from build123d import *

# Parameters (mm, degrees)
PAD001_DEPTH    = 30
POCKET002_DEPTH = 15
SKETCH010_R     = 2.951076
SKETCH010_W     = 16.720002
SKETCH010_H     = 13.459998
POCKET003_DEPTH = 5
SKETCH011_R     = 3.068583
SKETCH011_W     = 16.509998
SKETCH011_H     = 13.460002
POCKET004_DEPTH = 5


with BuildPart() as part:
    # Sketch008 → Pad001 (new body, symmetric)
    with BuildSketch(Plane.YZ):
        Polygon((-37.5, 10), (37.5, 10), (37.5, 30.376934), (-10.046035, 30.376934), align=None)
    extrude(amount=PAD001_DEPTH, both=True)

    # Sketch009 (on Face1 of Pad001) → Pocket002 (cut)
    with BuildSketch(Plane.YX.offset(-10)):
        with BuildLine():
            Line((-16.668194, 25.274987), (-16.668194, -26.160018))
            ThreePointArc((-16.668194, -26.160018), (-15.924248, -27.956072), (-14.128194, -28.700018))
            Line((-14.128194, -28.700018), (31.591806, -28.700018))
            ThreePointArc((31.591806, -28.700018), (33.387861, -27.956083), (34.131806, -26.160032))
            Line((34.131806, -26.160032), (34.131806, 25.909982))
            ThreePointArc((34.131806, 25.909982), (33.38786, 27.706037), (31.591806, 28.449982))
            Line((-13.493194, 28.449982), (31.591806, 28.449982))
            ThreePointArc((-13.493194, 28.449982), (-15.738253, 27.520045), (-16.668194, 25.274987))
        make_face()
    extrude(amount=-POCKET002_DEPTH, mode=Mode.SUBTRACT)

    # Sketch010 (on Face3 of Pocket002) → Pocket003 (cut)
    with BuildSketch(Plane(origin=(-30, 0, 0), x_dir=(0, 1, 0), z_dir=(-1, 0, 0))):
        with Locations((-9.634073, -10.729566)):
            Circle(SKETCH010_R)
        with Locations((19.018807, -14.92554)):
            Rectangle(SKETCH010_W, SKETCH010_H)
    extrude(amount=-POCKET003_DEPTH, mode=Mode.SUBTRACT)

    # Sketch011 (on Face14 of Pocket003) → Pocket004 (cut)
    with BuildSketch(Plane.YZ.offset(30)):
        with Locations((3.356387, 11.259916)):
            Circle(SKETCH011_R)
        with Locations((-9.699885, 11.221059)):
            Circle(SKETCH011_R)
        with Locations((18.913807, 14.92554)):
            Rectangle(SKETCH011_W, SKETCH011_H)
    extrude(amount=-POCKET004_DEPTH, mode=Mode.SUBTRACT)


solid = part.part
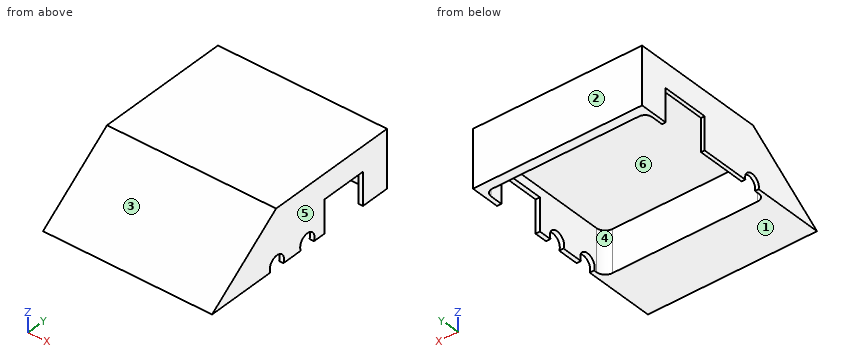
Input: part model. Units: mm. Frame: model coordinates. Face numbers are marked on the shaded views. A direction names the side the tool comes from. Coordinates: 2 decimals unless noted, no trailing zeros. Order: outer loops, then holes, each group sorted by start corner. A loop starts at its lowest first (then second) coordinate and runs counter-clockwise, first axis right, second up. Notation, with made-up numbers: M -26,-22.5 L -11,-22.5 A14 cw -11,-0.5 Z; hole C 8.25,-32 d4. An arc over 180 degrees is marked long. Answer in a Markdown table with one row per item.
(1) Section query D-D, the plane z = 15.75. Output: boundary loops of the cut face in (x, y).
Numbers:
| item | result |
|---|---|
| outline | M -30,-29.75 L 30,-29.75 L 30,10.66 L 28.45,10.66 L 28.45,-13.49 A3.18 cw 25.27,-16.67 L -26.16,-16.67 A2.54 cw -28.7,-14.13 L -28.7,10.66 L -30,10.66 Z; M -30,27.38 L -28.7,27.38 L -28.7,31.59 A2.54 cw -26.16,34.13 L 25.91,34.13 A2.54 cw 28.45,31.59 L 28.45,27.17 L 30,27.17 L 30,37.5 L -30,37.5 Z |
(2) Access query for the marked faces 5 and 6. Directions: +Z, -Z, +X, -X, +Y, -Y. A direction counts if a zero-diameter tool reaches every point of the face in a straight line with its end or side. Return the directions, or none.
Numbers:
| item | result |
|---|---|
| face 5 | +Z, -Z, +X, +Y, -Y |
| face 6 | -Z |
(3) Section query B-B, the plane z = 23. Output: boundary loops of the cut face in (x, y), plus the area to 3 significant figures.
Numbers:
| item | result |
|---|---|
| outline | M -30,-19.99 L 30,-19.99 L 30,37.5 L -30,37.5 Z; hole M -28.7,-14.13 A2.54 ccw -26.16,-16.67 L 25.27,-16.67 A3.18 ccw 28.45,-13.49 L 28.45,31.59 A2.54 ccw 25.91,34.13 L -26.16,34.13 A2.54 ccw -28.7,31.59 Z |
| area | 552 mm^2 |
(4) Material intervals for line 1 (X direction, y = 27, z = 22.5); line 2 (Z direction, x = 0.5, y = 32); line 3 (Y direction, x = 23, z = 11.75), sorted ascending. Write a range as [from, to].
Numbers:
| item | result |
|---|---|
| line 1 | x = [-30, -28.7], [28.45, 30] |
| line 2 | z = [25, 30.38] |
| line 3 | y = [-35.14, -16.67], [34.13, 37.5] |
(5) Section query A-A, the plane x = -25. Output: boundary loops of the cut face in (y, z).
Numbers:
| item | result |
|---|---|
| outline | M -37.5,10 L -16.67,10 L -16.67,25 L 34.13,25 L 34.13,10 L 37.5,10 L 37.5,30.38 L -10.05,30.38 Z |
(6) Draft query along Y for the marked faces 1, 2, 3 and 4. Return one class per face: pulls with the +Y half, pulls with the -Y half, needs draft (parallel to the pull), parting line crosses it, or undercut.
Numbers:
| item | result |
|---|---|
| face 1 | needs draft |
| face 2 | pulls with the +Y half |
| face 3 | pulls with the -Y half |
| face 4 | undercut |
(7) Contact query for flat-ended pins moving along their axis: pin 1 Ø10 at (x, y) = (-17.5, 11) entering from -Z; pin 2 Ø0.5 at (x, y) = (29, 19.5) entering from -Z; pin 3 Ø1.2 at (x, z) = (29.5, 17) entering from -Y. Output: stop coordinate, or through.
Numbers:
| item | result |
|---|---|
| pin 1 | stops at z = 25 |
| pin 2 | stops at z = 21.66 |
| pin 3 | stops at y = -28.88 |
(8) Section query C-C, the plane y = 22.5. Output: boundary loops of the cut face in (x, z), plus the area to 3 significant figures.
Numbers:
| item | result |
|---|---|
| outline | M -30,21.66 L -28.7,21.66 L -28.7,25 L 28.45,25 L 28.45,21.66 L 30,21.66 L 30,30.38 L -30,30.38 Z |
| area | 332 mm^2 |
